For this review, take the finished solid that the model builds, in its own axes (mm). A direction names the side the tool comes from. Give positions to 0.01 mm unless a question says otherwise; leave off trailing zeros. Write each loop counter-clockwise with the first axis right and the second up, starting at its lowest first coordinate (ties: lowest second). Pieces come first, ordered by that corner, then holes.
from build123d import *

# Parameters (mm, degrees)
F3_SIZE = 0.5
F4_SIZE = 3


with BuildPart() as f2:
    # F1 (on face) → F2 (revolve)
    with BuildSketch(Plane.XZ):
        Polygon((37.7653092146, 10.8646117151), (-5.6334966794, 10.8646117151), (-5.6334966794, 1.0394179262), (-6.8111736327, 1.0394179262), (-6.8111736327, -0.8785137325), (-5.6334966794, -0.8785137325), (-5.6334966794, -4.0582427464), (37.7653092146, -4.0582427464), align=None)
    revolve(axis=Axis((37.7653092146, 0, 3.4031844843), (0, 0, 1)))

    # F3
    f3_edges = [f2.edges().sort_by_distance(p)[0] for p in [
        (82.341792, 0, -0.878514),
    ]]
    chamfer(f3_edges, length=F3_SIZE)

    # F4
    f4_edges = [f2.edges().sort_by_distance(p)[0] for p in [
        (81.164115, 0, -4.058243),
    ]]
    chamfer(f4_edges, length=F4_SIZE)


solid = f2.part
(1) Tool access review of faces 1 (the flat face through (5, 29, -0.879)), 2 (the flat face through (80.5, 9.7, 1.039)), 3 (the flat face through (38, -1, -4.058)): name each direction out of +Z, -Z, +X, -X, +Y, -Y from which nothing blocks a thin tool from reaching the whole face with its end or side.
(2) For L1, parallel to Y at x = 39, z = 7; L2, parallel to Y at x = 5, z = 8; L3, parallel to X at y = 5, z = 1.75, list the stretches that pass through material, from the lowest coordinate up.
(3) We need section A-A (y = 0). Write out the cut boundary in (x, z), and give its area (3 significant figures).
(4) Clearance check with flat-ended pins moving along their axes: pin 1 Ø5 at (x, z) = (42, 9) entering from +Y; pin 2 Ø6 at (y, z) = (-12.5, -1.5) entering from +X; pin 3 Ø3 at (y, z) = (14, 5.5) entering from +X (3 decimals). State where each tip first meets the part, or that it passes through.
(5) We need section B-B (z = 2.75). Write out the cut boundary in (x, y), and give its area (3 significant figures).
The answers:
1. face 1: -Z
1. face 2: +Z
1. face 3: -Z, +X, -X, +Y, -Y
2. L1: y = -43.38 to 43.38
2. L2: y = -28.46 to 28.46
2. L3: x = -5.34 to 80.88
3. outline: (-6.81, -0.38) - (-6.31, -0.88) - (-5.63, -0.88) - (-5.63, -1.06) - (-2.63, -4.06) - (78.16, -4.06) - (81.16, -1.06) - (81.16, -0.88) - (81.84, -0.88) - (82.34, -0.38) - (82.34, 1.04) - (81.16, 1.04) - (81.16, 10.86) - (-5.63, 10.86) - (-5.63, 1.04) - (-6.81, 1.04) - close
3. area: 1,290 mm2
4. pin 1: stops at y = 43.36
4. pin 2: stops at x = 81.27
4. pin 3: stops at x = 79.325
5. outline: circle Ø86.8 at (37.77, 0)
5. area: 5,920 mm2
